Verification items for this drawing (mm, ordinates from the low corner). Round coordinates to 2 decimals unless told otherwise and drop trailing zeros. Order: outer loops, then holes, each group sorted by start corner. A loop starts at its lowest first (then second) coordinate and runs counter-clockwise, first axis right, second up.
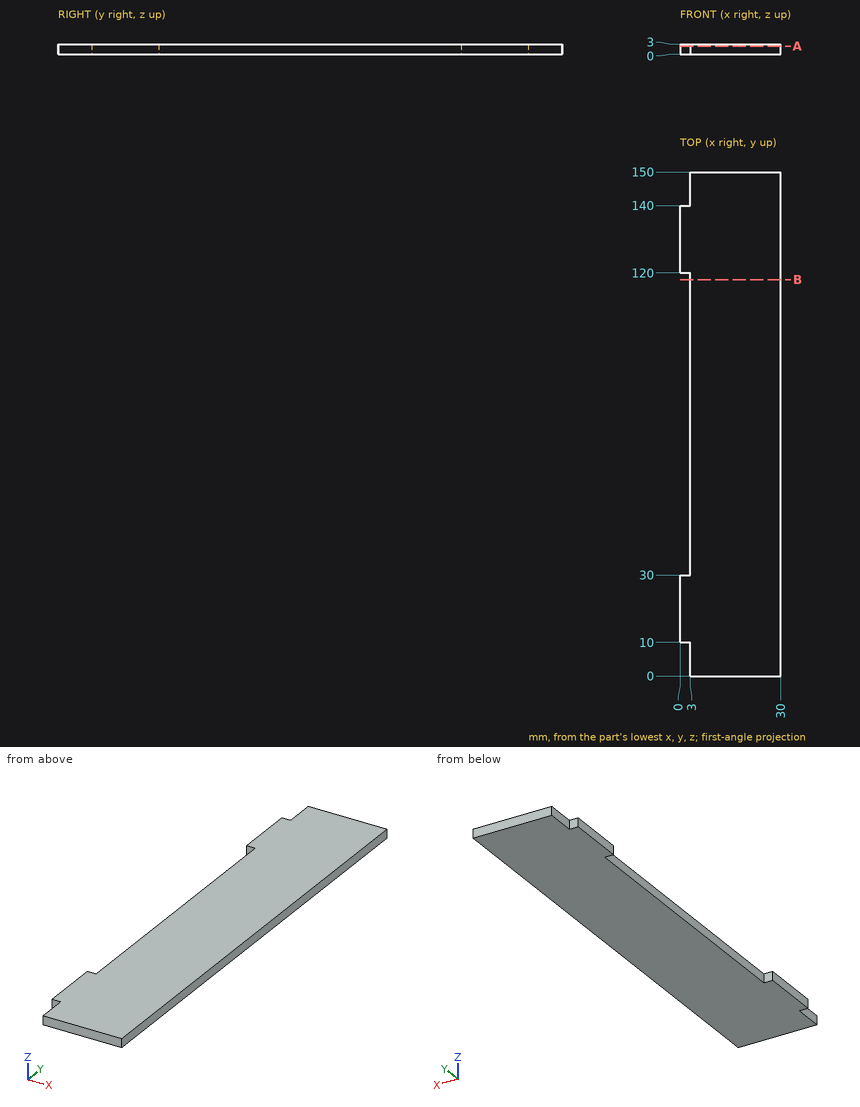
Item 1: Go/stop test with flat-tipped pins: P1, Ø5, axis at x = 20, y = 95.5, coming from the -Z side; P2, Ø1.5, axis at x = 1, z = 2, coming from the -Y side. Record where each tip stops, or that it passes through.
Answer:
P1: stops at z = 0
P2: stops at y = 10
Item 2: Sectioned sample at A-A (z = 2.4). Record the cut outline in (x, y).
Answer:
outline: (0, 10) - (3, 10) - (3, 0) - (30, 0) - (30, 150) - (3, 150) - (3, 140) - (0, 140) - (0, 120) - (3, 120) - (3, 30) - (0, 30) - close
Item 3: Sectioned sample at B-B (y = 118). Record the cut outline in (x, z), and give its area (3 significant figures).
Answer:
outline: (3, 0) - (30, 0) - (30, 3) - (3, 3) - close
area: 81.0 mm2
Item 4: Scan lines: line 1 along Y through (x, z) = (1.5, 2.25); line 2 along X through (y, z) = (83, 2.85). Record each from-to range of solid material in increasing order.
Answer:
line 1: y = 10 to 30, 120 to 140
line 2: x = 3 to 30
